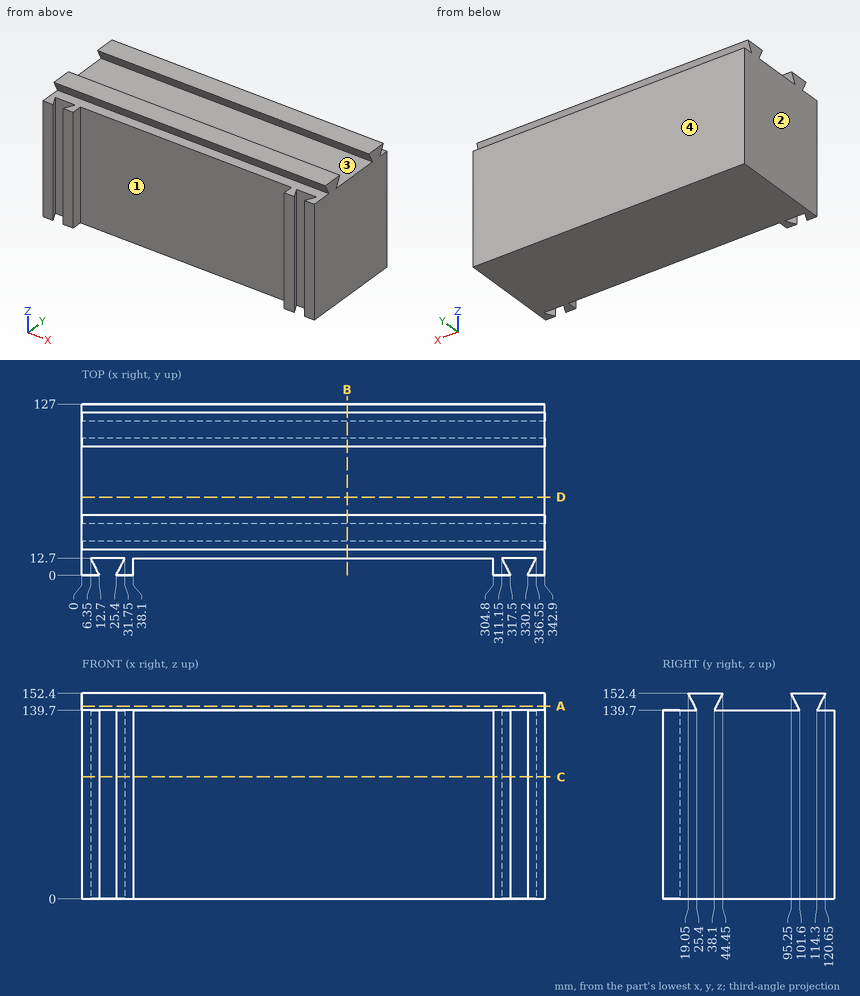
Geometry: see drawing. Coordinates: mm, zero at the bounding-box minimum. Round coordinates to 2 decimals unless told otherwise and drop trailing zeros. Loops run counter-clockwise (first coordinate to the right, second up) from the corner with the lowest first, then second, coordinate; pieces in that order, holes last. Notation, with made-up numbers: (-18, 26) - (4, 26) arc R17 cw to (4, 38) - close; hole circle Ø9 at (18, 48.5). An arc over 180 degrees is marked (long way). Use CSV: the item, a comma, the result in double quotes.
Q1. Pin query (flat end, axial travel): pin 1 Ø19 at (x, y) = (173, 61.5) entering from +Z; pin 2 Ø12 at (x, z) = (139.5, 35) entering from -Y. Return the tip coordinate at first contact, or that it passes through.
Reported:
pin 1,"z = 139.7"
pin 2,"y = 12.7"
Q2. Section query D-D, the plane y = 58. Output: boundary loops of the cut face in (x, z).
Reported:
outline,"(0, 0) - (342.9, 0) - (342.9, 139.7) - (0, 139.7) - close"
Q3. Ray query, line 1 along Y through (x, z) = (57, 33); line 2 along Z through (x, y) = (134, 65); line 3 along Y through (x, z) = (15.5, 144.5). Return the intervals inside material, ascending.
Reported:
line 1,"12.7 to 127"
line 2,"0 to 139.7"
line 3,"23 to 40.5, 99.2 to 116.7"
Q4. Section query C-C, the plane z = 90.5. Output: boundary loops of the cut face in (x, y), then the cut area to 3 significant figures.
Reported:
outline,"(0, 0) - (12.7, 0) - (6.35, 12.7) - (31.75, 12.7) - (25.4, 0) - (38.1, 0) - (38.1, 12.7) - (304.8, 12.7) - (304.8, 0) - (317.5, 0) - (311.15, 12.7) - (336.55, 12.7) - (330.2, 0) - (342.9, 0) - (342.9, 127) - (0, 127) - close"
area,"39,700 mm^2"
Q5. Section query B-B, the plane x = 196.5. Output: boundary loops of the cut face in (y, z).
Reported:
outline,"(12.7, 0) - (127, 0) - (127, 139.7) - (114.3, 139.7) - (120.65, 152.4) - (95.25, 152.4) - (101.6, 139.7) - (38.1, 139.7) - (44.45, 152.4) - (19.05, 152.4) - (25.4, 139.7) - (12.7, 139.7) - close"
Q6. Section query A-A, the plane z = 143. Output: boundary loops of the cut face in (x, y), then the cut area to 3 significant figures.
Reported:
outline,"(0, 23.75) - (342.9, 23.75) - (342.9, 39.75) - (0, 39.75) - close; (0, 99.95) - (342.9, 99.95) - (342.9, 115.95) - (0, 115.95) - close"
area,"11,000 mm^2"
Q7. Mould query, pull axis Y, two halves, no side actions, for the marked faces 1, 2, 3 and 4. Classes: pulls with the +Y half, pulls with the -Y half, needs draft (parallel to the pull), parting line crosses it, or undercut.
Reported:
face 1,"pulls with the -Y half"
face 2,"needs draft"
face 3,"undercut"
face 4,"pulls with the +Y half"
